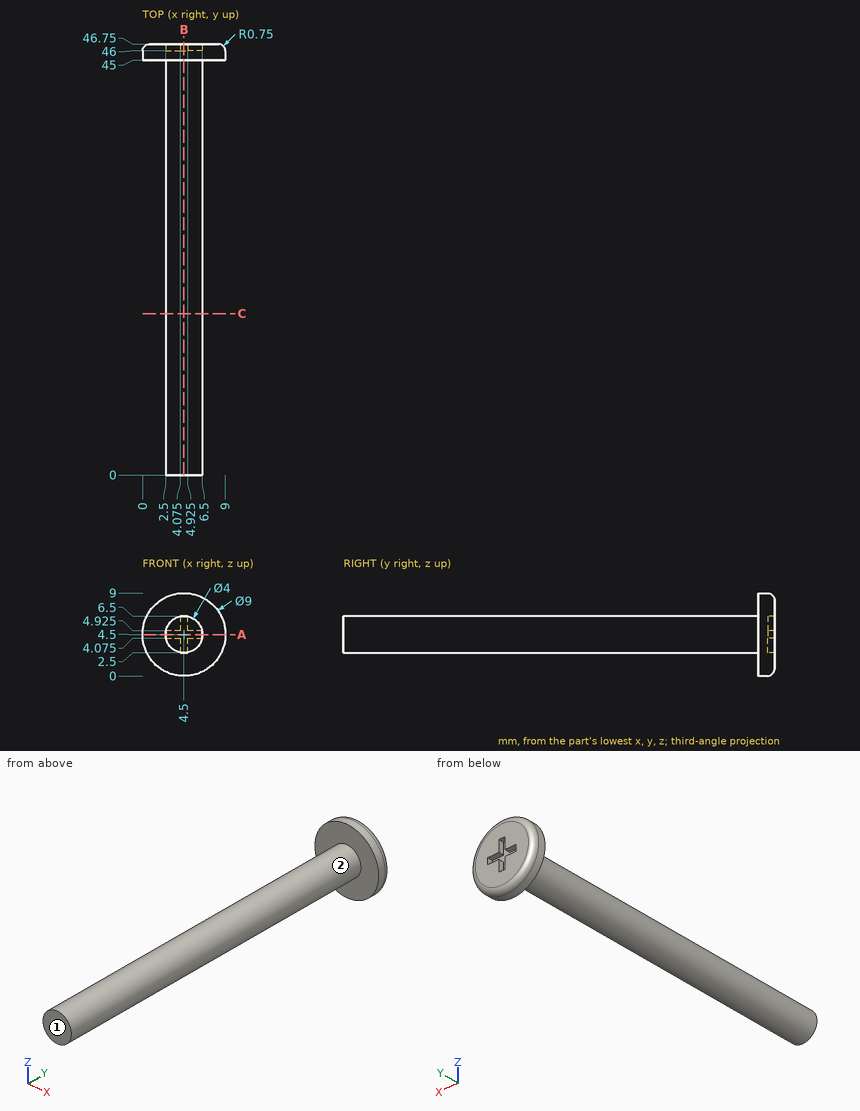
Could you check a few things on this drawing? It's one solid part, dimensions in mm from its lowest x, y, z. A direction names the side the tool comes from. Give positions to 0.01 mm unless a question says otherwise; leave off trailing zeros. Order: outer loops, then holes, each group sorted by start corner. A loop starts at its lowest first (then second) coordinate and runs counter-clockwise, first axis right, second up. Notation, with made-up numbers: M 32.5,41.25 L 53.5,41.25 A26 cw 53.5,58.25 Z; hole C 64,16.5 d2. An arc over 180 degrees is marked long. Use one line per item in the form item = value. Start each with the question number.
Item 1: For the marked faces 1 and 2, which set-ups out of +Z, -Z, +X, -X, +Y, -Y let a thin tool reach every point of the face, with its end or its side?
Item 2: If we section it at C-C (y = 17.5): Write out the boundary of the cut face in (x, z), then the cut area to 3 significant figures.
Item 3: If I drill on line 1 along Y through (x, z) = (3, 1); line 2 along X through (y, z) = (17, 6), over which ranges is the centre line in solid material (lowest first)?
Item 4: If we section it at A-A (z = 4.5): Write out the boundary of the cut face in (x, y).
Item 5: Will these pins go through, and if not, where does the flat tip stop? pin 1 Ø1.5 at (x, z) = (4.5, 5) entering from +Y; pin 2 Ø0.8 at (x, y) = (6, 46.5) entering from +Z; pin 3 Ø1.5 at (x, y) = (3, 14.5) entering from +Z; pin 4 Ø3 at (y, z) = (16.5, 1.5) entering from +X.
Item 6: If we section it at B-B (x = 4.5): Write out the boundary of the cut face in (y, z).
Outcome:
q1.face_1 = +Z, -Z, +X, -X, -Y
q1.face_2 = -Y
q2.outline = C 4.5,4.5 d4
q2.area = 12.6 mm2
q3.line_1 = 45 to 46.75
q3.line_2 = 3.18 to 5.82
q4.outline = M 0,45 L 2.5,45 L 2.5,0 L 6.5,0 L 6.5,45 L 9,45 L 9,46 A0.75 ccw 8.25,46.75 L 6.5,46.75 L 6.5,46 L 2.5,46 L 2.5,46.75 L 0.75,46.75 A0.75 ccw 0,46 Z
q5.pin_1 = 46.75
q5.pin_2 = 8.8
q5.pin_3 = 6.35
q5.pin_4 = 5.82
q6.outline = M 0,2.5 L 45,2.5 L 45,0 L 46,0 A0.75 ccw 46.75,0.75 L 46.75,2.5 L 46,2.5 L 46,6.5 L 46.75,6.5 L 46.75,8.25 A0.75 ccw 46,9 L 45,9 L 45,6.5 L 0,6.5 Z
